Could you check a few things on this model? Use its own coordinates, in mm. A direction names the side the tool comes from. Give positions to 0.01 mm unless a question says otherwise; leave off trailing zeros. Order: outer loops, then holes, each group sorted by start corner. A loop starts at its lowest first (then second) coordinate and runs counter-clockwise, first axis right, second up.
Autodesk Inventor part; units mm, degrees
ref_plane "YZ Plane" through (0, 0, 0) normal (1, 0, 0) x (0, 1, 0)
ref_plane "XZ Plane" through (0, 0, 0) normal (0, 1, 0) x (-1, 0, 0)
ref_plane "XY Plane" through (0, 0, 0) normal (0, 0, 1) x (1, 0, 0)
sketch "Skizze1" plane through (0, 0, 0) normal (0, 0, 1) x (1, 0, 0)
  line L0 (0, 0) -> (15, 0)
  arc A0 (20, -1) -> (15, 0) centre (15, -13) ccw
  line L1 (20, -1) -> (45, -11.4167)
  arc A1 (50, -18.9167) -> (45, -11.4167) centre (41.875, -18.9167) ccw
  line L2 (50, -18.9167) -> (50, -41.6467)
  arc A2 (50, -41.6467) -> (55, -46.6467) centre (55, -41.6467) ccw
  line L3 (55, -46.6467) -> (60, -46.6467)
  line L4 (60, -46.6467) -> (66.5, -46.6467)
  line L5 (0, 0) -> (-6.5, 0)
  point P0 (57.5, -46.6467)
  dimension "d0" = 15
  dimension "d1" = 20
  dimension "d2" = 1
  dimension "d3" = 45
  dimension "d4" = 5
  dimension "d5" = 22.73
  dimension "d6" = 5
  dimension "d7" = 5
  dimension "d20" = 46.6467
  dimension "d22" = 6.5
  dimension "d23" = 6.5
sketch "Skizze2" plane through (0, 0, 0) normal (1, 0, 0) x (0, 1, 0)
  circle A0 centre (0, 0) radius 2
  dimension "d16" = 4
sweep "Sweeping1" add profiles "Skizze2" path "Skizze1"
equation "\"d22\" = d23"
properties part number "front iron bar"
Item 1: Please list where these lines run through material, in increasing order: line 1 along Y through (x, z) = (55, -0.5); line 2 along X through (y, z) = (-20, -1.6); line 3 along Y through (x, z) = (19, -0.9).
Findings:
line 1: y = -48.58 to -44.71
line 2: x = 48.8 to 51.2
line 3: y = -2.52 to 1.23
Item 2: Imagine slicing it at A-A on y = -23. List the corners of the cut face in (x, z) for me, then the cut area to 3 significant figures.
Findings:
outline: circle Ø4 at (50, 0)
area: 12.6 mm2
Item 3: For faces 1 (the flat face through (-6.5, 0, 0)), 2 (the cylindrical face through (51.847, -30.441, -0.766)), which set-ups out of +Z, -Z, +X, -X, +Y, -Y let a thin tool reach every point of the face, with its end or its side?
Findings:
face 1: +Z, -Z, -X, +Y, -Y
face 2: none
Item 4: For pin 1 (12 mm diameter, centred on x = 56.5, y = -9, fed in from -Z); pin 2 (2 mm diameter, centred on y = -27, z = 1.5, fed in from -X); pin 3 (1.5 mm diameter, centred on y = -9, z = 0, fed in from +X), each with a flat end and sliding along its axis, tell me the tip position at first contact or that it passes through.
Findings:
pin 1: passes through
pin 2: stops at x = 48.06
pin 3: stops at x = 46.17
